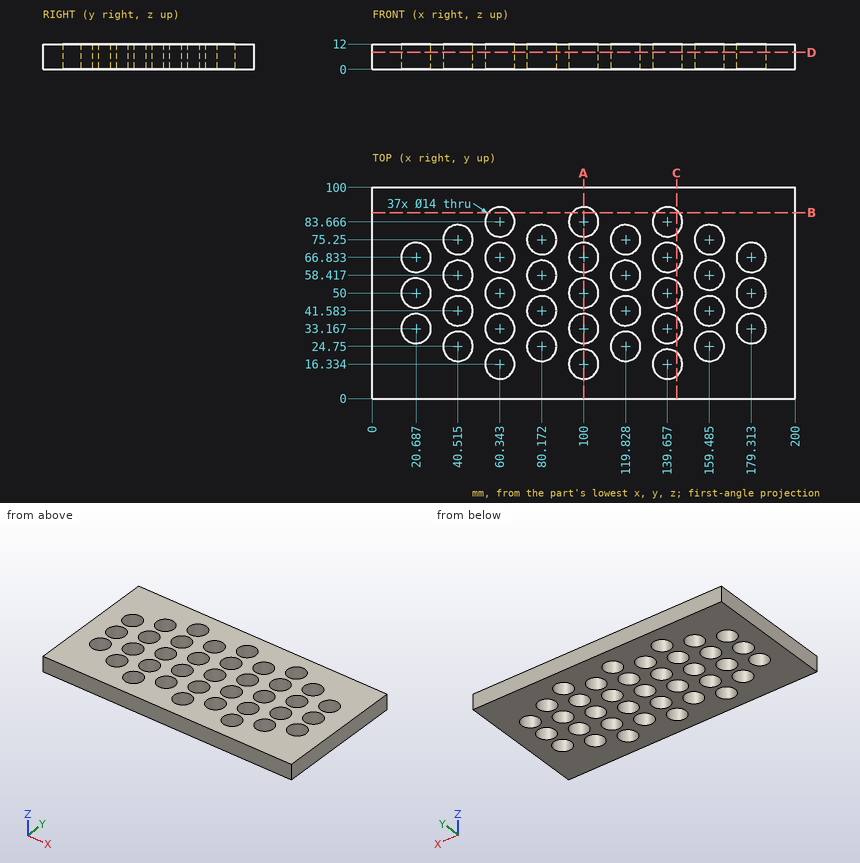
Could you check a few things on this drawing? It's one solid part, dimensions in mm from its lowest x, y, z. Round coordinates to 2 decimals unless told otherwise and drop trailing zeros. Order: outer loops, then holes, each group sorted by start corner. A loop starts at its lowest first (then second) coordinate and runs counter-clockwise, first axis right, second up. Notation, with made-up numbers: M -40,89.5 L -13,89.5 A30 ccw -13,124.5 Z; hole C 53,42.25 d9. An arc over 180 degrees is marked long. One line per question, with ' | ' between items.
1) Imagine slicing it at C-C, the plane x = 144. Write out the boundary of the cut face in (y, z).
Checked values:
outline: M 0,0 L 10.84,0 L 10.84,12 L 0,12 Z; M 21.82,0 L 27.68,0 L 27.68,12 L 21.82,12 Z; M 38.66,0 L 44.51,0 L 44.51,12 L 38.66,12 Z; M 55.49,0 L 61.34,0 L 61.34,12 L 55.49,12 Z; M 72.32,0 L 78.18,0 L 78.18,12 L 72.32,12 Z; M 89.16,0 L 100,0 L 100,12 L 89.16,12 Z
2) Imagine slicing it at D-D, the plane z = 8. Count the separate pieces of the cut face and the enclosed holes in it, plus the area to 3 significant figures.
Checked values:
separate pieces: 1 | enclosed holes: 37 | area: 14,300 mm²
3) Imagine slicing it at A-A, the plane x = 100. Write out the boundary of the cut face in (y, z), plus the area to 3 significant figures.
Checked values:
outline: M 0,0 L 9.33,0 L 9.33,12 L 0,12 Z; M 23.33,0 L 26.17,0 L 26.17,12 L 23.33,12 Z; M 40.17,0 L 43,0 L 43,12 L 40.17,12 Z; M 57,0 L 59.83,0 L 59.83,12 L 57,12 Z; M 73.83,0 L 76.67,0 L 76.67,12 L 73.83,12 Z; M 90.67,0 L 100,0 L 100,12 L 90.67,12 Z | area: 360 mm²
4) Imagine slicing it at B-B, the plane y = 88. Write out the boundary of the cut face in (x, z).
Checked values:
outline: M 0,0 L 54.85,0 L 54.85,12 L 0,12 Z; M 65.84,0 L 94.5,0 L 94.5,12 L 65.84,12 Z; M 105.5,0 L 134.16,0 L 134.16,12 L 105.5,12 Z; M 145.15,0 L 200,0 L 200,12 L 145.15,12 Z
5) I need wall thicknesses on line 1 (X direction, y = 41, z = 1); line 2 (Y direction, x = 100, z = 4); line 3 (X direction, y = 33.5, z = 4.5) (1 decimal). Which ranges of each line are inside material? Lowest first, please.
Checked values:
line 1: x = 0 to 33.54, 47.49 to 73.2, 87.15 to 112.85, 126.8 to 152.51, 166.46 to 200 | line 2: y = 0 to 9.33, 23.33 to 26.17, 40.17 to 43, 57 to 59.83, 73.83 to 76.67, 90.67 to 100 | line 3: x = 0 to 13.7, 27.7 to 53.4, 67.3 to 93, 107 to 132.7, 146.6 to 172.3, 186.3 to 200
6) I'm going to push a flat-ended pin straight in: pin 1 Ø11 at (x, y) = (20.69, 50) entering from +Z. Where does the tip first touch, or does it pass through?
Checked values:
pin 1: passes through
